Study the drawing (mm; zero at the part's minimum x, y, z) and answer. Round coordinates to 2 decimals unless told otherwise and drop trailing zeros. Write each loop counter-clockwise with the first axis right and the second up, starting at its lowest first coordinate (ties: lowest second). Pieces come first, ordered by that corner, then holes. Notation, with made-up numbers: (88, -7) - (94, -7) arc R13 ccw to (94, 4) - close; hole circle Ø2 at (58, 18). An arc over 180 degrees is marked (long way). Return JSON: item names as keys, results as strings. Group by question number.
(1) Find the intervals of material crossed by line 1 along X through (y, z) = (9, 102); line 2 along Z through (x, y) = (64.5, 5.75); line 3 along X through (y, z) = (7.25, 54), in increasing order. Write a range as [from, to].
(2) Section C-C, the plane x = 35.5 is taken. Write down the section's boundary in (y, z).
(3) Section B-B, the plane y = 3.5 is taken. Write down the section's boundary in (x, z), then the cut area to 3 significant figures.
(4) Section A-A, the plane z = 102 is taken. Write down the section's boundary in (x, y), then the cut area to 3 significant figures.
(5) Each of these flat-tipped pins is pushed along its axis until it touches: pin 1 (2 mm diameter, centred on x = 44, y = 6.5, fed in from -Z); pin 2 (5.5 mm diameter, centred on x = 17.5, z = 56, fed in from -Y). Where does it stop, or does it pass through?
(6) Section D-D, the plane z = 53 is taken. Write down the section's boundary in (x, y).
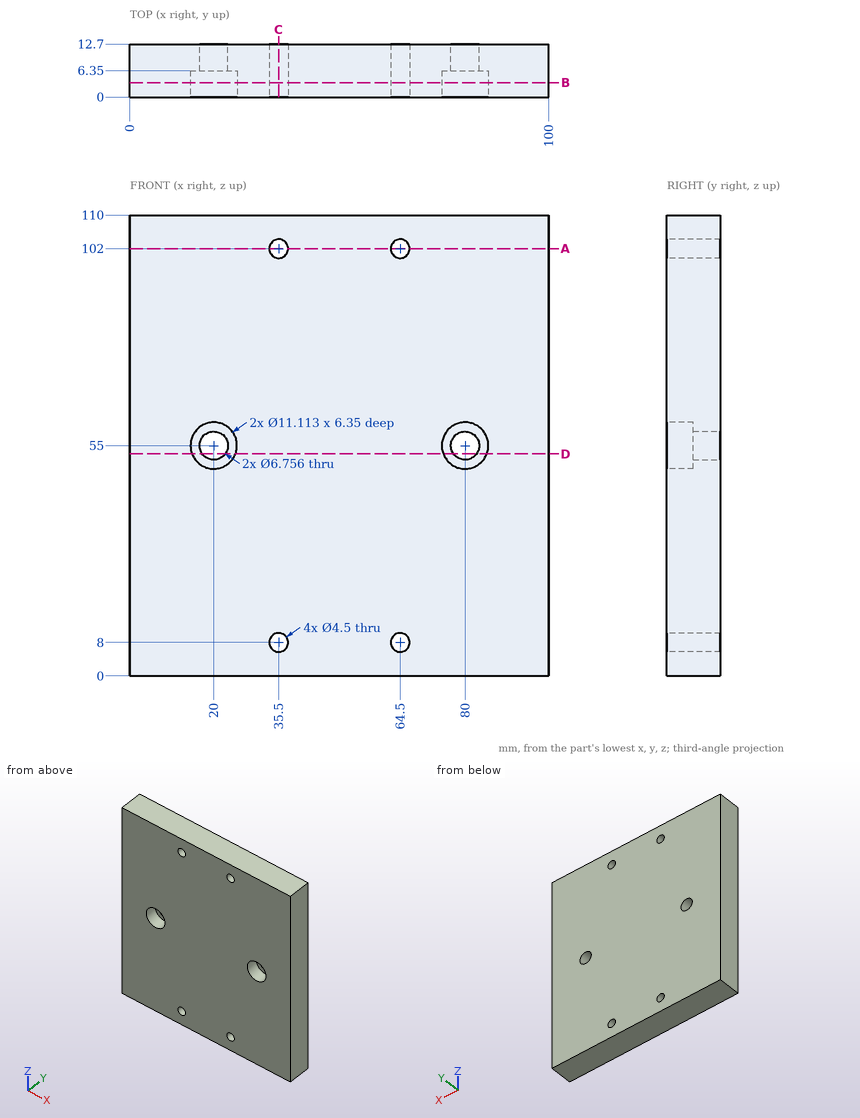
Working result:
{
 "1": {"line 1": "x = [0, 33.25], [37.75, 62.25], [66.75, 100]", "line 2": "z = [0, 5.75], [10.25, 99.75], [104.25, 110]", "line 3": "x = [0, 16.77], [23.23, 76.77], [83.23, 100]"},
 "2": {"outline": "(0, 0) - (12.7, 0) - (12.7, 5.75) - (0, 5.75) - close; (0, 10.25) - (12.7, 10.25) - (12.7, 99.75) - (0, 99.75) - close; (0, 104.25) - (12.7, 104.25) - (12.7, 110) - (0, 110) - close"},
 "3": {"outline": "(0, 0) - (100, 0) - (100, 110) - (0, 110) - close; hole circle Ø11.11 at (20, 55); hole circle Ø4.5 at (35.5, 8); hole circle Ø4.5 at (35.5, 102); hole circle Ø4.5 at (64.5, 8); hole circle Ø4.5 at (64.5, 102); hole circle Ø11.11 at (80, 55)", "area": "10,700 mm^2"},
 "4": {"outline": "(0, 0) - (33.25, 0) - (33.25, 12.7) - (0, 12.7) - close; (37.75, 0) - (62.25, 0) - (62.25, 12.7) - (37.75, 12.7) - close; (66.75, 0) - (100, 0) - (100, 12.7) - (66.75, 12.7) - close", "area": "1,160 mm^2"},
 "5": {"pin 1": "stops at z = 0", "pin 2": "stops at y = 6.35"},
 "6": {"outline": "(0, 0) - (14.82, 0) - (14.82, 6.35) - (17.28, 6.35) - (17.28, 12.7) - (0, 12.7) - close; (22.72, 6.35) - (25.18, 6.35) - (25.18, 0) - (74.82, 0) - (74.82, 6.35) - (77.28, 6.35) - (77.28, 12.7) - (22.72, 12.7) - close; (82.72, 6.35) - (85.18, 6.35) - (85.18, 0) - (100, 0) - (100, 12.7) - (82.72, 12.7) - close"}
}
